from build123d import *

# Parameters (mm, degrees)
SKETCH1_R           = 1.75
BOSS_EXTRUDE1_DEPTH = 3
SKETCH2_R           = 3.5
CUT_EXTRUDE1_DEPTH  = 1
FILLET1_R           = 1


with BuildPart() as part:
    # Sketch1 → Boss-Extrude1 (new body)
    with BuildSketch(Plane.XY):
        with BuildLine():
            Line((-5.845671476, 25.875), (-25.331243061, -7.875))
            ThreePointArc((-25.331243061, -7.875), (-25.331243061, -14.625), (-19.485571585, -18))
            Line((-19.485571585, -18), (-1.5, -18))
            Line((-1.5, -18), (-1.5, -7.858116823))
            ThreePointArc((-1.5, -7.858116823), (-8, 0), (-1.5, 7.858116823))
            Line((-1.5, 7.858116823), (-1.5, 18))
            Line((-1.5, 18), (1.5, 18))
            Line((1.5, 18), (1.5, 7.858116823))
            ThreePointArc((1.5, 7.858116823), (6.164414003, 5.099019514), (8, 0))
            ThreePointArc((8, 0), (6.164414003, -5.099019514), (1.5, -7.858116823))
            Line((1.5, -7.858116823), (1.5, -18))
            Line((1.5, -18), (19.485571585, -18))
            ThreePointArc((19.485571585, -18), (25.331243061, -14.625), (25.331243061, -7.875))
            Line((25.331243061, -7.875), (5.845671476, 25.875))
            ThreePointArc((5.845671476, 25.875), (0, 29.25), (-5.845671476, 25.875))
        make_face()
        with Locations((-19.485571585, -11.25)):
            Circle(SKETCH1_R, mode=Mode.SUBTRACT)
        with Locations((19.485571585, -11.25)):
            Circle(SKETCH1_R, mode=Mode.SUBTRACT)
        with Locations((0, 22.5)):
            Circle(SKETCH1_R, mode=Mode.SUBTRACT)
    extrude(amount=BOSS_EXTRUDE1_DEPTH)

    # Sketch2 → Cut-Extrude1 (cut)
    with BuildSketch(Plane.XY.offset(3)):
        with Locations((0, 22.5)):
            Circle(SKETCH2_R)
        with Locations((19.485571585, -11.25)):
            Circle(SKETCH2_R)
        with Locations((-19.485571585, -11.25)):
            Circle(SKETCH2_R)
    extrude(amount=-CUT_EXTRUDE1_DEPTH, mode=Mode.SUBTRACT)

    # Fillet1
    fillet1_edges = [part.edges().sort_by_distance(p)[0] for p in [
        (-3.5, 22.5, 3),
        (15.985571585, -11.25, 3),
        (-22.985571585, -11.25, 3),
    ]]
    fillet(fillet1_edges, radius=FILLET1_R - 0.0001)  # a hair under: the kernel refuses the full size


solid = part.part
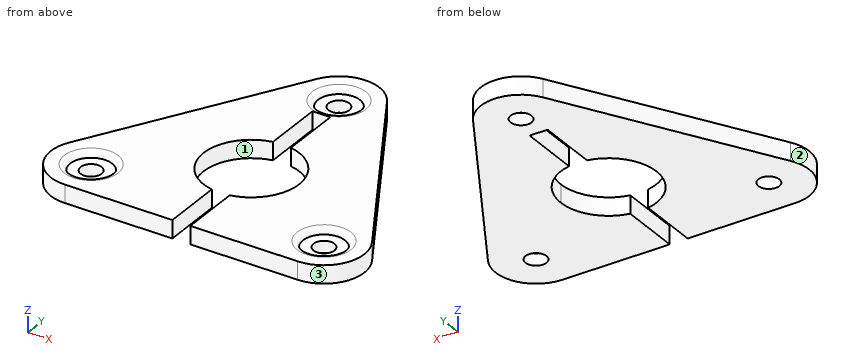
Model file for the job. Use its own axes, mm. Face numbers are marked on the shaded views. Give positions to 0.01 mm unless a question says otherwise; leave off trailing zeros. Loops run counter-clockwise (first coordinate to the right, second up) from the corner with the lowest first, then second, coordinate; pieces in that order, holes last.
1) Saw through at D-D (y = -11.25). Count the separate pieces of the cut face and the enclosed holes in it, plus the area to 3 significant figures.
2) Wall check: line 1 (X direction, y = -11.25, z = 0.5); line 2 (Y direction, x = 0, z = 1.35); line 3 (X direction, y = -14.5, z = 2.45). Give the ranges that are in metal, low to high.
3) Flat gauge pins, fed straight in: pin 1 Ø0.9 at (y, z) = (14.5, 1) entering from +X; pin 2 Ø1 at (y, z) = (5, 2.5) entering from -X; pin 3 Ø1.5 at (y, z) = (12, 2) entering from -X. Where does each tip first touch, or does it go through?
4) Saw through at C-C (y = -3). Write the cut outline in (x, z), plus the area to 3 significant figures.
5) Saw through at B-B (z = 1.25). Write the cut outline in (x, y) (3 decimals), plus the area to 3 significant figures.
6) Pull direction X, two halves, no side cores. Call the marked faces 1, 2 and 3: +X half, -X half, draft (parallel to the pull), parting line (faces both ways), or undercut.
Answer block:
1. separate pieces: 4
1. enclosed holes: 0
1. area: 120 mm2
2. line 1: x = -26.24 to -21.24, -17.74 to -1.5, 1.5 to 17.74, 21.24 to 26.24
2. line 2: y = 18 to 20.75, 24.25 to 29.25
2. line 3: x = -25.4 to -21.05, -17.92 to -1.5, 1.5 to 17.92, 21.05 to 25.4
3. pin 1: stops at x = 12.67
3. pin 2: stops at x = -18.19
3. pin 3: stops at x = -14.29
4. outline: (-22.52, 0) - (-7.42, 0) - (-7.42, 3) - (-22.52, 3) - close; (7.42, 0) - (22.52, 0) - (22.52, 3) - (7.42, 3) - close
4. area: 90.6 mm2
5. outline: (-25.331, -7.875) arc R6.75 ccw to (-19.486, -18) - (-1.5, -18) - (-1.5, -7.858) arc R8 cw to (-1.5, 7.858) - (-1.5, 18) - (1.5, 18) - (1.5, 7.858) arc R8 cw to (1.5, -7.858) - (1.5, -18) - (19.486, -18) arc R6.75 ccw to (25.331, -7.875) - (5.846, 25.875) arc R6.75 ccw to (-5.846, 25.875) - close; hole circle Ø3.5 at (-19.486, -11.25); hole circle Ø3.5 at (0, 22.5); hole circle Ø3.5 at (19.486, -11.25)
5. area: 1,300 mm2
6. face 1: undercut
6. face 2: -X half
6. face 3: +X half
